Geometry check sheet. Reference: the model listing, model coordinates, mm. Face numbers are marked on the shaded views. Coordinates: 2 decimals unless noted, no trailing zeros. Write each loop counter-clockwise with the first axis right and the second up, starting at its lowest first coordinate (ties: lowest second). Pieces come first, ordered by that corner, then holes. Notation, with made-up numbers: (5.5, 70) -> (34.5, 70) arc R30 cw to (34.5, 109) -> close; hole circle Ø7 at (27, -16.5). An arc over 180 degrees is marked (long way). Use a Markdown table: item, result.
```python
from build123d import *

# Parameters (mm, degrees)
SKETCH2_R          = 0.85
CUT_EXTRUDE1_DEPTH = 1.1


with BuildPart() as part:
    # Sketch1 → Revolve1 (revolve)
    with BuildSketch(Plane.XY, mode=Mode.PRIVATE) as revolve1_sk:
        Polygon((0, -10.15), (0, 10.15), (0.9, 10.15), (0.9, 3.15), (3.05, 3.15), (3.05, 2.55), (12.1, 2.55), (12.1, -9.65), (11.9, -9.65), (11.9, -9.05), (2.85, -9.05), (2.85, -10.15), align=None)
    revolve(revolve1_sk.sketch.rotate(Axis((0, -11.843181818, 0), (0, 1, 0)), 90), axis=Axis((0, -11.843181818, 0), (0, 1, 0)))

    # Sketch2 → Cut-Extrude1 (cut)
    with BuildSketch(Plane(origin=(0, 2.55, 0), x_dir=(1, 0, 0), z_dir=(0, 1, 0))):
        with Locations(Location((-8.25, 0, 0), (0, 0, 270))):
            Circle(SKETCH2_R)
        with Locations(Location((-4.125, 7.144709581, 0), (0, 0, 270))):
            Circle(SKETCH2_R)
        with Locations(Location((4.125, 7.144709581, 0), (0, 0, 270))):
            Circle(SKETCH2_R)
        with Locations(Location((8.25, 0, 0), (0, 0, 270))):
            Circle(SKETCH2_R)
        with Locations(Location((4.125, -7.144709581, 0), (0, 0, 270))):
            Circle(SKETCH2_R)
        with Locations(Location((-4.125, -7.144709581, 0), (0, 0, 270))):
            Circle(SKETCH2_R)
    extrude(amount=-CUT_EXTRUDE1_DEPTH, mode=Mode.SUBTRACT)


solid = part.part
```
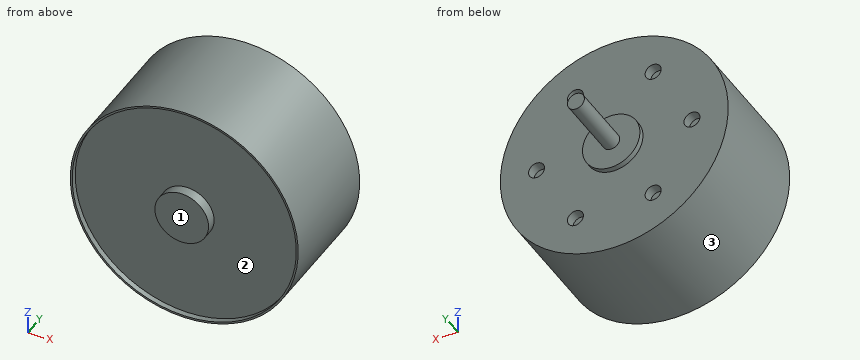
Item 1: Depth check by flat-ended pin: P1, Ø2, axis at x = -8.25, z = 0, coming from the +Y side; P2, Ø1.5, axis at x = 8.25, z = 0, coming from the -Y side; P3, Ø1, axis at x = -4.12, z = 7.14, coming from the +Y side. Enter the tip coordinate at first touch or a pass-through.
Answer block:
| item | result |
|---|---|
| P1 | stops at y = 2.55 |
| P2 | stops at y = -9.05 |
| P3 | stops at y = 1.45 |
Item 2: Section check D-D on y = -5. Record the boundary of the cut face in (x, z), then the cut area to 3 significant figures.
Answer block:
| item | result |
|---|---|
| outline | circle Ø24.2 at (0, 0) |
| area | 460 mm^2 |
Item 3: Thickness scan on L1, parallel to X at y = 1.7, z = 0; L2, parallel to X at y = -9.35, z = 0; L3, parallel to X at y = -2.25, z = 0.25. Record the ranges inside material, lowest first. Write a range as [from, to].
Answer block:
| item | result |
|---|---|
| L1 | x = [-12.1, -9.1], [-7.4, 7.4], [9.1, 12.1] |
| L2 | x = [-12.1, -11.9], [-2.85, 2.85], [11.9, 12.1] |
| L3 | x = [-12.1, 12.1] |
Item 4: Section check B-B on z = -1.5. Record the boundary of the cut face in (x, y).
Answer block:
| item | result |
|---|---|
| outline | (-12.01, -9.65) -> (-11.81, -9.65) -> (-11.81, -9.05) -> (-2.42, -9.05) -> (-2.42, -10.15) -> (2.42, -10.15) -> (2.42, -9.05) -> (11.81, -9.05) -> (11.81, -9.65) -> (12.01, -9.65) -> (12.01, 2.55) -> (2.66, 2.55) -> (2.66, 3.15) -> (-2.66, 3.15) -> (-2.66, 2.55) -> (-12.01, 2.55) -> close |
Item 5: Mould release check, pull along X, two halves, no side actions. Record for the marked faces 1, 2 and 3: +X half, -X half, draft (parallel to the pull), parting line (faces both ways), or undercut.
Answer block:
| item | result |
|---|---|
| face 1 | draft |
| face 2 | undercut |
| face 3 | parting line |
Item 6: Section check A-A on x = 0. Record the boundary of the cut face in (y, z), then the cut area to 3 significant figures.
Answer block:
| item | result |
|---|---|
| outline | (-10.15, -2.85) -> (-9.05, -2.85) -> (-9.05, -11.9) -> (-9.65, -11.9) -> (-9.65, -12.1) -> (2.55, -12.1) -> (2.55, -3.05) -> (3.15, -3.05) -> (3.15, -0.9) -> (10.15, -0.9) -> (10.15, 0.9) -> (3.15, 0.9) -> (3.15, 3.05) -> (2.55, 3.05) -> (2.55, 12.1) -> (-9.65, 12.1) -> (-9.65, 11.9) -> (-9.05, 11.9) -> (-9.05, 2.85) -> (-10.15, 2.85) -> close |
| area | 303 mm^2 |
Item 7: Section check C-C on y = 2. Record the boundary of the cut face in (x, z) (3 decimals).
Answer block:
| item | result |
|---|---|
| outline | circle Ø24.2 at (0, 0); hole circle Ø1.7 at (-8.25, 0); hole circle Ø1.7 at (-4.125, -7.145); hole circle Ø1.7 at (-4.125, 7.145); hole circle Ø1.7 at (4.125, -7.145); hole circle Ø1.7 at (4.125, 7.145); hole circle Ø1.7 at (8.25, 0) |
